from build123d import *

# Parameters (mm, degrees)
SKETCH1_R           = 45
BOSS_EXTRUDE1_DEPTH = 16
SKETCH2_R           = 7.5
CUT_EXTRUDE1_DEPTH  = 66.620118866
SKETCH3_R           = 6.700020908
CUT_EXTRUDE2_DEPTH  = 13.617825
CIRPATTERN1_START   = 2.382174647
CIRPATTERN1_DEPTH   = 13.617825353


# Read off the part's stored shape, not the designer's step: CirPattern1
with BuildPart() as part:
    # Sketch1 → Boss-Extrude1 (new body)
    with BuildSketch(Plane(origin=(0, 0, 0), x_dir=(1, 0, 0), z_dir=(0, 1, 0))):
        with Locations(Location((0, 0, 0), (0, 0, 270))):
            Circle(SKETCH1_R)
    extrude(amount=BOSS_EXTRUDE1_DEPTH)

    # Sketch2 → Cut-Extrude1 (cut, through all)
    with BuildSketch(Plane(origin=(0, 0, 0), x_dir=(1, 0, 0), z_dir=(0, 1, 0))):
        with Locations(Location((0, 0, 0), (0, 0, 270))):
            Circle(SKETCH2_R)
    extrude(amount=CUT_EXTRUDE1_DEPTH, mode=Mode.SUBTRACT)

    # Sketch3 → Cut-Extrude2 (cut)
    with BuildSketch(Plane(origin=(0, 16, 0), x_dir=(1, 0, 0), z_dir=(0, 1, 0))):
        with Locations((-10.430928244, 0)):
            Circle(SKETCH3_R)
    extrude(amount=-CUT_EXTRUDE2_DEPTH, mode=Mode.SUBTRACT)

    # CirPattern1 outline → CirPattern1 (cut)
    with BuildSketch(Plane(origin=(0, 0, 0), x_dir=(1, 0, 0), z_dir=(0, 1, 0)).offset(CIRPATTERN1_START)):
        with BuildLine():
            ThreePointArc((-5.759985164, -4.803391605), (-9.656933393, -6.655164321), (-13.874844674, -5.74714884))
            ThreePointArc((-13.874844674, -5.74714884), (-12.113410314, -12.113410314), (-5.74714884, -13.874844674))
            ThreePointArc((-5.74714884, -13.874844674), (0, -17.130949152), (5.74714884, -13.874844674))
            ThreePointArc((5.74714884, -13.874844674), (12.113410314, -12.113410314), (13.874844674, -5.74714884))
            ThreePointArc((13.874844674, -5.74714884), (17.130949152, 0), (13.874844674, 5.74714884))
            ThreePointArc((13.874844674, 5.74714884), (12.113410314, 12.113410314), (5.74714884, 13.874844674))
            ThreePointArc((5.74714884, 13.874844674), (0, 17.130949152), (-5.74714884, 13.874844674))
            ThreePointArc((-5.74714884, 13.874844674), (-12.113410314, 12.113410314), (-13.874844674, 5.74714884))
            ThreePointArc((-13.874844674, 5.74714884), (-9.656933393, 6.655164321), (-5.759985164, 4.803391605))
            ThreePointArc((-5.759985164, 4.803391605), (7.5, 0), (-5.759985164, -4.803391605))
        make_face()
    extrude(amount=CIRPATTERN1_DEPTH, mode=Mode.SUBTRACT)


solid = part.part
Build history of the part. All positions in model axes, mm. A direction names the side the tool comes from. Coordinates: 2 decimals unless noted, no trailing zeros. Order: outer loops, then holes, each group sorted by start corner. A loop starts at its lowest first (then second) coordinate and runs counter-clockwise, first axis right, second up. Notation, with made-up numbers: (26, 17) -> (63, 17) arc R18 ccw to (63, 40) -> close; hole circle Ø9 at (8.5, 57). An arc over 180 degrees is marked (long way). One line per item, written item: value.
(1) Mould opens along Z. For faces 1 (the flat face through (-19, 16, -1)), 2 (the cylindrical face through (-17.235, 7.888, 41.569)), 3 (the cylindrical face through (-12.045, 9.096, -12.181)) say: pulls with the +Z half, pulls with the -Z half, needs draft (parallel to the pull), parting line crosses it, or undercut.
Checked values:
face 1: needs draft
face 2: parting line crosses it
face 3: undercut
(2) Slice it at B-B, the plane x = 0. List the corners of the cut face in (y, z).
Checked values:
outline: (0, -45) -> (16, -45) -> (16, -17.13) -> (2.38, -17.13) -> (2.38, -7.5) -> (0, -7.5) -> close; (0, 7.5) -> (2.38, 7.5) -> (2.38, 17.13) -> (16, 17.13) -> (16, 45) -> (0, 45) -> close
(3) Slice it at C-C, the plane y = 8.75. List the corners of the cut face in (x, z).
Checked values:
outline: circle Ø90 at (0, 0); hole (-13.87, -5.75) arc R6.7 ccw to (-5.75, -13.87) arc R6.7 ccw to (5.75, -13.87) arc R6.7 ccw to (13.87, -5.75) arc R6.7 ccw to (13.87, 5.75) arc R6.7 ccw to (5.75, 13.87) arc R6.7 ccw to (-5.75, 13.87) arc R6.7 ccw to (-13.87, 5.75) arc R6.7 ccw to start
(4) Drop flat-ended pins along their axis: pin 1 Ø1.5 at (x, y) = (-33.5, 10.5) entering from -Z; pin 2 Ø8 at (y, z) = (6, -24) entering from +X; pin 3 Ø3 at (x, z) = (-31, 8.5) entering from -Y; pin 4 Ø5 at (y, z) = (7.5, 17.5) entering from -X. Give the stop position or say it passes through.
Checked values:
pin 1: z = -30.86
pin 2: x = 40.31
pin 3: y = 0
pin 4: x = -42.43
(5) Slice it at A-A, the plane z = 0. List the corners of the cut face in (x, y), plus the area to 3 significant figures.
Checked values:
outline: (-45, 0) -> (-7.5, 0) -> (-7.5, 2.38) -> (-17.13, 2.38) -> (-17.13, 16) -> (-45, 16) -> close; (7.5, 0) -> (45, 0) -> (45, 16) -> (17.13, 16) -> (17.13, 2.38) -> (7.5, 2.38) -> close
area: 938 mm2
(6) Slice it at D-D, the plane x = -11. List the corners of the cut face in (y, z).
Checked values:
outline: (0, -43.63) -> (16, -43.63) -> (16, -13.01) -> (2.38, -13.01) -> (2.38, 13.01) -> (16, 13.01) -> (16, 43.63) -> (0, 43.63) -> close
(7) Tool access for faces 4 (the cylindrical face through (-2.87, 1.17, 6.93)), 5 (the cylindrical face through (-0.1, 9.1, 17.13)): list every direction of +Z, -Z, +X, -X, +Y, -Y with a clear straight run to the whole face (end or side of a thin tool).
Checked values:
face 4: +Y, -Y
face 5: +Y
(8) Probe line 1 (Z direction, x = 0.5, y = 6); line 2 (X direction, y = 0.8, z = 0); line 3 (X direction, y = 9.75, z = 0). List the from-to ranges inside material, lowest first. Write a range as [from, to].
Checked values:
line 1: [-45, -17.11], [17.11, 45]
line 2: [-45, -7.5], [7.5, 45]
line 3: [-45, -17.13], [17.13, 45]
